from build123d import *

# Parameters (mm, degrees)
BOSS_EXTRUDE1_DEPTH = 5.08


with BuildPart() as part:
    # Sketch1 → Boss-Extrude1 (new body)
    with BuildSketch(Plane(origin=(0, 0, 0), x_dir=(1, 0, 0), z_dir=(0, 1, 0))):
        Polygon((-2.579450384, -0.091335292), (-2.579450384, 2.43268731), (2.524046381, 2.43268731), (2.524046381, -0.091335292), (2.524046381, -2.615357894), (-2.579450384, -2.615357894), align=None)
        with BuildLine():
            Line((-1.559427547, -0.599335292), (-0.867135524, -0.599335292))
            ThreePointArc((-0.867135524, -0.599335292), (-0.706426639, -0.782360667), (-0.508, -0.923613994))
            Line((-0.508, -0.923613994), (-0.508, -1.5621))
            ThreePointArc((-0.508, -1.5621), (0, -2.0701), (0.508, -1.5621))
            Line((0.508, -1.5621), (0.508, -0.923613994))
            ThreePointArc((0.508, -0.923613994), (0.706426639, -0.782360667), (0.867135524, -0.599335292))
            Line((0.867135524, -0.599335292), (1.559427547, -0.599335292))
            ThreePointArc((1.559427547, -0.599335292), (2.067427547, -0.091335292), (1.559427547, 0.416664708))
            Line((1.559427547, 0.416664708), (0.968254786, 0.416664708))
            ThreePointArc((0.968254786, 0.416664708), (0.7804367, 0.708551598), (0.508, 0.923613994))
            Line((0.508, 0.923613994), (0.508, 1.5621))
            ThreePointArc((0.508, 1.5621), (0, 2.0701), (-0.508, 1.5621))
            Line((-0.508, 1.5621), (-0.508, 0.923613994))
            ThreePointArc((-0.508, 0.923613994), (-0.7804367, 0.708551598), (-0.968254786, 0.416664708))
            Line((-0.968254786, 0.416664708), (-1.559427547, 0.416664708))
            ThreePointArc((-1.559427547, 0.416664708), (-2.067427547, -0.091335292), (-1.559427547, -0.599335292))
        make_face(mode=Mode.SUBTRACT)
    extrude(amount=BOSS_EXTRUDE1_DEPTH)


solid = part.part
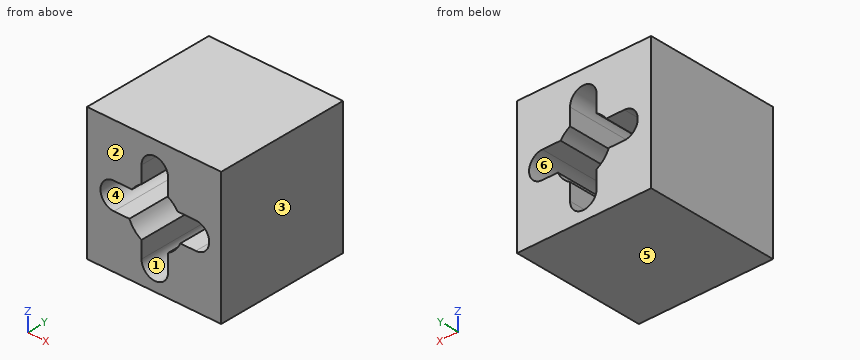
Could you check a few things on this model? Use its own coordinates, in mm. Face numbers are marked on the shaded views. A direction names the side the tool comes from. Give positions to 0.01 mm unless a question says otherwise; leave off trailing zeros. Order: outer loops, then holes, each group sorted by start corner. A loop starts at its lowest first (then second) coordinate and runs counter-clockwise, first axis right, second up.
Item 1: For the marked faces 5 and 6, which set-ups out of +Z, -Z, +X, -X, +Y, -Y let a thin tool reach every point of the face, with its end or its side?
Item 2: If we mould it in two halves opening along X, with no side actions, what happens to the marked faces 1, 2, 3 and 4? For each: pulls with the +X half, pulls with the -X half, needs draft (parallel to the pull), parting line crosses it, or undercut.
Item 3: I need wall thicknesses on line 1 (Z direction, x = 0.6, y = 0.9); line 2 (Z direction, x = 1, y = 4); line 3 (X direction, y = 0.8, z = -1.55). Which ranges of each line are inside material? Lowest first, please.
Item 4: If we section it at A-A, the plane x = 0: Write out the boundary of the cut face in (y, z).
Item 5: If we section it at C-C, the plane y = 1.2: Write out the boundary of the cut face in (x, z), plus the area to 3 significant figures.
Item 6: If we section it at B-B, the plane z = 1.1: Write out the boundary of the cut face in (x, y).
Values:
1. face 5: -Z, +X, -X, +Y, -Y
1. face 6: +Y, -Y
2. face 1: undercut
2. face 2: needs draft
2. face 3: pulls with the +X half
2. face 4: undercut
3. line 1: z = -2.43 to -0.87, 0.87 to 2.62
3. line 2: z = -2.43 to -0.42, 0.6 to 2.62
3. line 3: x = -2.58 to -0.51, 0.51 to 2.52
4. outline: (0, -2.43) - (5.08, -2.43) - (5.08, -2.07) - (0, -2.07) - close; (0, 2.07) - (5.08, 2.07) - (5.08, 2.62) - (0, 2.62) - close
5. outline: (-2.58, -2.43) - (2.52, -2.43) - (2.52, 2.62) - (-2.58, 2.62) - close; hole (-1.56, -0.42) - (-0.97, -0.42) arc R1.05 ccw to (-0.51, -0.92) - (-0.51, -1.56) arc R0.51 ccw to (0.51, -1.56) - (0.51, -0.92) arc R1.05 ccw to (0.97, -0.42) - (1.56, -0.42) arc R0.51 ccw to (1.56, 0.6) - (0.87, 0.6) arc R1.05 ccw to (0.51, 0.92) - (0.51, 1.56) arc R0.51 ccw to (-0.51, 1.56) - (-0.51, 0.92) arc R1.05 ccw to (-0.87, 0.6) - (-1.56, 0.6) arc R0.51 ccw to start
5. area: 18.4 mm2
6. outline: (-2.58, 0) - (-0.51, 0) - (-0.51, 5.08) - (-2.58, 5.08) - close; (0.51, 0) - (2.52, 0) - (2.52, 5.08) - (0.51, 5.08) - close
